Autodesk Inventor part; units mm, degrees
ref_plane "YZ Plane" through (0, 0, 0) normal (1, 0, 0) x (0, 1, 0)
ref_plane "XZ Plane" through (0, 0, 0) normal (0, 1, 0) x (-1, 0, 0)
ref_plane "XY Plane" through (0, 0, 0) normal (0, 0, 1) x (1, 0, 0)
sketch "Sketch1" plane through (0, 0, 0) normal (0, 1, 0) x (-1, 0, 0)
  line L0 (120, 36) -> (-120, 36)
  line L1 (-120, 36) -> (-120, -36)
  line L2 (-120, -36) -> (120, -36)
  line L3 (120, -36) -> (120, 36)
  line L4 (120, 36) -> (-120, -36) construction
  line L5 (-120, 36) -> (120, -36) construction
  line L6 (125, 41) -> (-125, 41)
  line L7 (-125, 41) -> (-125, -41)
  line L8 (-125, -41) -> (125, -41)
  line L9 (125, -41) -> (125, 41)
  point P0 (0, 0)
  dimension "d0" = 72
  dimension "d1" = 240
  dimension "d2" = 5
extrude "Extrusion1" add sketch "Sketch1" along normal blind 10 contours L3 L2 L1 L0
extrude "Extrusion2" add sketch "Sketch1" along normal blind 50
sketch "Sketch2" plane through (-125, 0, 41) normal (0, 0, 1) x (1, 0, 0)
  circle A0 centre (5, 5) radius 3.2
  line L0 (0, 0) -> (0, 50)
  line L1 (0, 0) -> (250, 0)
  point P0 (125, 0)
  dimension "d9" = 6.4
  dimension "d22" = 5
  dimension "d23" = 5
extrude "Extrusion3" cut sketch "Sketch2" against normal through all
sketch "Sketch3" plane through (0, 0, 0) normal (0, -1, 0) x (1, 0, 0)
  point P0 (0, 0)
properties part number "GiveBox"
Geometry: final body of the model. Coordinates: model frame, mm. A direction names the side the tool comes from. Coordinates: 2 decimals unless noted, no trailing zeros. Loops run counter-clockwise (first coordinate to the right, second up) from the corner with the lowest first, then second, coordinate; pieces in that order, holes last. Notation, with made-up numbers: (-1.75, -33) - (52.25, -33) arc R38 ccw to (52.25, 6) - close; hole circle Ø4 at (64, 15.25). An arc over 180 degrees is marked (long way). One line per question, with ' | ' between items. Start each with the question number.
(1) Reachability of faces 1 (the flat face through (19.1, 50, -36.3)), 2 (the flat face through (-2, 30, 36)) from +Z, -Z, +X, -X, +Y, -Y: full face, straight path, thin tool, end or side. Return the list, or none.
(2) Cut plane A-A on y = 5. Output: boundary loops of the cut face in (x, z).
(3) Cut plane B-B on y = 17.5. Output: boundary loops of the cut face in (x, z), and give its area (3 significant figures).
(4) First-contact query: pin 1 (5 mm diameter, centred on x = -120, y = 5, fed in from +Z); pin 2 (1.5 mm diameter, centred on x = 14, z = 14, fed in from +Y). Flat tips, straight axial feed; report the tip coordinate or a pass-through.
(5) Cut plane D-D on x = -66. Output: boundary loops of the cut face in (y, z).
(6) Cut plane C-C on z = -15. Output: boundary loops of the cut face in (x, y), and give its area (3 significant figures).
(7) Ray query, L1, parallel to X at y = 46.5, z = 17.5; L2, parallel to Z at x = -109.5, y = 44; L3, parallel to Y at x = 67, z = 32. Return the intervals inside material, ascending. Write a range as from..to.
(8) Draft query along Z for faces 3 (the flat face through (-120, 30, -1)), 4 (the flat face through (-2, 25, 41)), 5 (the flat face through (2, 0, 1)), 6 (the flat face through (120, 30, 1)). Return one class per face: +Z half, -Z half, draft (parallel to the pull), parting line (faces both ways), or undercut.
Here are the results:
1) face 1: +Z, -Z, +X, -X, +Y | face 2: +Y
2) outline: (-125, -41) - (-123.2, -41) - (-123.2, 41) - (-125, 41) - close; (-116.8, -41) - (125, -41) - (125, 41) - (-116.8, 41) - close
3) outline: (-125, -41) - (125, -41) - (125, 41) - (-125, 41) - close; hole (-120, -36) - (120, -36) - (120, 36) - (-120, 36) - close | area: 3,220 mm²
4) pin 1: through | pin 2: y = 10
5) outline: (0, -41) - (50, -41) - (50, -36) - (10, -36) - (10, 36) - (50, 36) - (50, 41) - (0, 41) - close
6) outline: (-125, 0) - (125, 0) - (125, 50) - (120, 50) - (120, 10) - (-120, 10) - (-120, 50) - (-125, 50) - close; hole circle Ø6.4 at (-120, 5) | area: 2,870 mm²
7) L1: -125..-120, 120..125 | L2: -41..-36, 36..41 | L3: 0..10
8) face 3: undercut | face 4: +Z half | face 5: draft | face 6: undercut
